Check sheet for the modelled part. Datum: model origin and axes. Units: mm. A direction names the side the tool comes from. Give positions to 0.01 mm unless a question says otherwise; leave off trailing zeros. Order: outer loops, then holes, each group sorted by start corner. A loop starts at its lowest first (then second) coordinate and runs counter-clockwise, first axis right, second up.
from build123d import *

# Parameters (mm, degrees)
F0_W     = 185.788676
F0_H     = 167.966946
F1_DEPTH = 101.6
F2_W     = 71.583546
F2_H     = 55.591479
F3_DEPTH = 635
F4_W     = 161.412612
F4_H     = 155.637712
F5_DEPTH = 1270
F6_R     = 23.160944
F7_DEPTH = 635


with BuildPart() as f1:
    # F0 (on Top) → F1 (new body)
    with BuildSketch(Plane.XY):
        Rectangle(F0_W, F0_H)
    extrude(amount=F1_DEPTH)

    # F2 (on Front) → F3 (cut, symmetric)
    with BuildSketch(Plane.XZ):
        with Locations((0, 76.723866)):
            Rectangle(F2_W, F2_H)
    extrude(amount=F3_DEPTH, both=True, mode=Mode.SUBTRACT)

    # F4 (on face) → F5 (cut)
    with BuildSketch(Plane(origin=(0, 0, 0), x_dir=(1, 0, 0), z_dir=(0, 0, -1))):
        Rectangle(F4_W, F4_H)
    extrude(amount=-F5_DEPTH, mode=Mode.SUBTRACT)

    # F6 (on Right) → F7 (cut, symmetric)
    with BuildSketch(Plane.YZ):
        with Locations((0, 46.262771)):
            Circle(F6_R)
    extrude(amount=F7_DEPTH, both=True, mode=Mode.SUBTRACT)


solid = f1.part
1) Section check B-B, the plane y = 0. Record the cut outline in (x, z), then the cut area to 3 significant figures.
Recorded:
outline: (-92.89, 0) - (-80.71, 0) - (-80.71, 23.1) - (-92.89, 23.1) - close; (-92.89, 69.42) - (-80.71, 69.42) - (-80.71, 101.6) - (-92.89, 101.6) - close; (80.71, 0) - (92.89, 0) - (92.89, 23.1) - (80.71, 23.1) - close; (80.71, 69.42) - (92.89, 69.42) - (92.89, 101.6) - (80.71, 101.6) - close
area: 1,350 mm2
2) Section check D-D, the plane y = 49.5. Record the cut outline in (x, z).
Recorded:
outline: (-92.89, 0) - (-80.71, 0) - (-80.71, 101.6) - (-92.89, 101.6) - close; (80.71, 0) - (92.89, 0) - (92.89, 101.6) - (80.71, 101.6) - close
3) Section check C-C, the plane z = 85. Record the cut outline in (x, y).
Recorded:
outline: (-92.89, -83.98) - (-35.79, -83.98) - (-35.79, -77.82) - (-80.71, -77.82) - (-80.71, 77.82) - (-35.79, 77.82) - (-35.79, 83.98) - (-92.89, 83.98) - close; (35.79, -83.98) - (92.89, -83.98) - (92.89, 83.98) - (35.79, 83.98) - (35.79, 77.82) - (80.71, 77.82) - (80.71, -77.82) - (35.79, -77.82) - close
4) Material ranges on L1, parallel to X at y = -64, z = 86; L2, parallel to Y at x = 65, z = 54; L3, parallel to Z at x = 86.25, y = 0, recorded low to high.
Recorded:
L1: x = -92.89 to -80.71, 80.71 to 92.89
L2: y = -83.98 to -77.82, 77.82 to 83.98
L3: z = 0 to 23.1, 69.42 to 101.6
5) Depth check by flat-ended pin: pin 1 Ø1.8 at (x, y) = (-7, -79.5) entering from +Z. Enter the tip coordinate at first touch or a pass-through.
Recorded:
pin 1: stops at z = 48.93
6) Set-up check for faces 4 (the face through (-1, -81, 48.928)), 5 (the face through (83, 0, 101.6)), 6 (the face through (80.706, 18.4, 61.4)): record each of +Z, -Z, +X, -X, +Y, -Y from which the full face is reachable in a straight line by a thin tool's end or side.
Recorded:
face 4: +Z, +Y, -Y
face 5: +Z, +X, -X, +Y, -Y
face 6: +Z, -Z
7) Section check A-A, the plane x = 25. Record the cut outline in (y, z), then the cut area to 3 significant figures.
Recorded:
outline: (-83.98, 0) - (-77.82, 0) - (-77.82, 48.93) - (-83.98, 48.93) - close; (77.82, 0) - (83.98, 0) - (83.98, 48.93) - (77.82, 48.93) - close
area: 603 mm2
8) Draft check along Y on faces 1 (the face through (0, 81, 0)), 2 (the face through (-1, -83.983, 39)), 3 (the face through (86.886, 12.451, 65.792)). Enter one of: +Y half, -Y half, draft (parallel to the pull), parting line (faces both ways), or undercut.
Recorded:
face 1: draft
face 2: -Y half
face 3: undercut
